Here's how the part is built. I have some questions about the finished solid (model axes, mm). Round coordinates to 2 decimals unless told otherwise and drop trailing zeros. Put each result on its own line as item: value. Start each with the question number.
1. For pin 1 (4 mm diameter, centred on x = 37, y = -211, fed in from -Z), with a flat end and sliding along its axis, tell me the tip position at first contact or that it passes through.
2. We'd pull the mould along Y, two halves only. Please class faces 1 (the face through (195, -245, 2)), 2 (the face through (195, 95, 2)), 3 (the face through (86.315, -66.596, 2.535)): +Y half, -Y half, draft (parallel to the pull), parting line (faces both ways), or undercut.
3. Suppose I cut it at A-A (z = 3.6). Count the separate pieces of the cut face and the enclosed holes in it, then the cut area to 3 significant figures.
4. I need wall thicknesses on probe 1 along Y at (x, z) = (-90, 1.65); probe 2 along Y at (x, z) = (150, 3.3); probe 3 along X at (y, z) = (-223, 1.9). Which ranges of each line are inside material? Lowest first, please. Write a range as from..to.
```python
from build123d import *

# Parameters (mm, degrees)
F0_W      = 400
F0_H      = 350
F1_DEPTH  = 5
F2_R      = 17
F3_DEPTH  = 25
F5_D      = 3.3
F7_D      = 3.3
F9_D      = 3.3
F11_DEPTH = 25
F13_D     = 3.3
F15_D     = 3.3
F17_D     = 2.5
F18_D     = 5
F20_D     = 2.5
F22_D     = 6.8
F23_SIZE  = 10


with BuildPart() as f1:
    # F0 (on Top) → F1 (new body)
    with BuildSketch(Plane.XY):
        with Locations((0, -75)):
            Rectangle(F0_W, F0_H)
    extrude(amount=F1_DEPTH)

    # F2 (on face) → F3 (cut)
    with BuildSketch(Plane.XY.offset(5)):
        with Locations((-90, -50)):
            Circle(F2_R)
        with Locations((90, -50)):
            Circle(F2_R)
    extrude(amount=-F3_DEPTH, mode=Mode.SUBTRACT)

    # F5 (through all)
    with Locations(Plane.XY.offset(5)):
        with Locations((-90, -72), (-68, -50), (-90, -28), (-112, -50), (68, -50), (90, -72), (112, -50), (90, -28)):
            Hole(F5_D / 2)

    # F7 (through all)
    with Locations(Plane.XY.offset(5)):
        with Locations((-6, -225), (6, -225), (6, -240), (-6, -240)):
            Hole(F7_D / 2)

    # F9 (through all)
    with Locations(Plane(origin=(0, 0, 0), x_dir=(1, 0, 0), z_dir=(0, 0, -1))):
        with Locations((-145, 225), (-145, 195), (35, 195), (35, 225)):
            Hole(F9_D / 2)

    # F10 (on face) → F11 (cut)
    with BuildSketch(Plane.XY.offset(5)):
        with BuildLine():
            Line((-101, -230), (-101, -200))
            ThreePointArc((-101, -200), (-106, -195), (-111, -200))
            Line((-111, -200), (-111, -230))
            ThreePointArc((-111, -230), (-106, -235), (-101, -230))
        make_face()
        with BuildLine():
            Line((69, -200), (69, -230))
            ThreePointArc((69, -230), (74, -235), (79, -230))
            Line((79, -230), (79, -200))
            ThreePointArc((79, -200), (74, -195), (69, -200))
        make_face()
    extrude(amount=-F11_DEPTH, mode=Mode.SUBTRACT)

    # F13 (through all)
    with Locations(Plane(origin=(0, 0, 0), x_dir=(1, 0, 0), z_dir=(0, 0, -1))):
        with Locations((-102, -20), (-102, 0), (150, 0), (150, -20)):
            Hole(F13_D / 2)

    # F15 (through all)
    with Locations(Plane(origin=(0, 0, 0), x_dir=(1, 0, 0), z_dir=(0, 0, -1))):
        with Locations((-150, 20), (-150, 90), (150, 90), (150, 20)):
            Hole(F15_D / 2)

    # F17 (through all)
    with Locations(Plane(origin=(0, 0, 0), x_dir=(1, 0, 0), z_dir=(0, 0, -1))):
        with Locations((-75, 180), (-67, 180), (67, 180), (75, 180)):
            Hole(F17_D / 2)

    # F18 (through all)
    with Locations(Plane(origin=(0, 0, 0), x_dir=(1, 0, 0), z_dir=(0, 0, -1))):
        with Locations((-37, 180), (37, 180)):
            Hole(F18_D / 2)

    # F20 (through all)
    with Locations(Plane(origin=(0, 0, 0), x_dir=(1, 0, 0), z_dir=(0, 0, -1))):
        with Locations((-167.8194442075, -4.4897614533), (-12.1805557925, -4.4897614533), (-90, 145), (12.1805557925, -4.4897614533), (167.8194442075, -4.4897614533), (90, 145)):
            Hole(F20_D / 2)

    # F22 (through all)
    with Locations(Plane.XY.offset(5)):
        with Locations((-40, -87), (-40, -155), (40, -155), (40, -87)):
            Hole(F22_D / 2)

    # F23
    f23_edges = [f1.edges().sort_by_distance(p)[0] for p in [
        (-200, -250, 2.5),
        (200, -250, 2.5),
        (200, 100, 2.5),
        (-200, 100, 2.5),
    ]]
    chamfer(f23_edges, length=F23_SIZE)


solid = f1.part
```
Verdict:
1. pin 1: stops at z = 0
2. face 1: -Y half
2. face 2: +Y half
2. face 3: undercut
3. separate pieces: 1
3. enclosed holes: 44
3. area: 137,000 mm^2
4. probe 1: y = -250..-146.25, -143.75..-73.65, -70.35..-67, -33..-29.65, -26.35..100
4. probe 2: y = -250..-91.65, -88.35..-21.65, -18.35..-1.65, 1.65..18.35, 21.65..100
4. probe 3: x = -200..-111, -101..69, 79..200
